Could you check a few things on this drawing? It's one solid part, dimensions in mm from its lowest x, y, z. Round coordinates to 2 decimals unless told otherwise and drop trailing zeros. Loops run counter-clockwise (first coordinate to the right, second up) from the corner with the lowest first, then second, coordinate; pieces in that order, holes last. Notation, with made-up numbers: (44, 60.25) -> (65, 60.25) arc R34 cw to (65, 90.25) -> close; hole circle Ø8 at (-29.75, 75.25). An arc over 180 degrees is marked (long way). Put each result on its own line as item: value. Start each with the question number.
1. Imagine slicing it at C-C, the plane y = 17.25. Please give me the cut outline in (x, z), and give its area (3 significant figures).
2. Imagine slicing it at D-D, the plane z = 23. Please give me the cut outline in (x, y).
3. Imagine slicing it at A-A, the plane x = 66.04. Please give me the cut outline in (y, z), and give its area (3 significant figures).
4. Imagine slicing it at B-B, the plane z = 19.05. Please give me the cut outline in (x, y), and give its area (3 significant figures).
5. I need wall thicknesses on line 1 (Z direction, x = 17.5, y = 23.25); line 2 (Z direction, x = 70.5, y = 1.5); line 3 (X direction, y = 15, z = 2). Which ranges of each line are inside material? Lowest first, please. Write a range as [from, to].
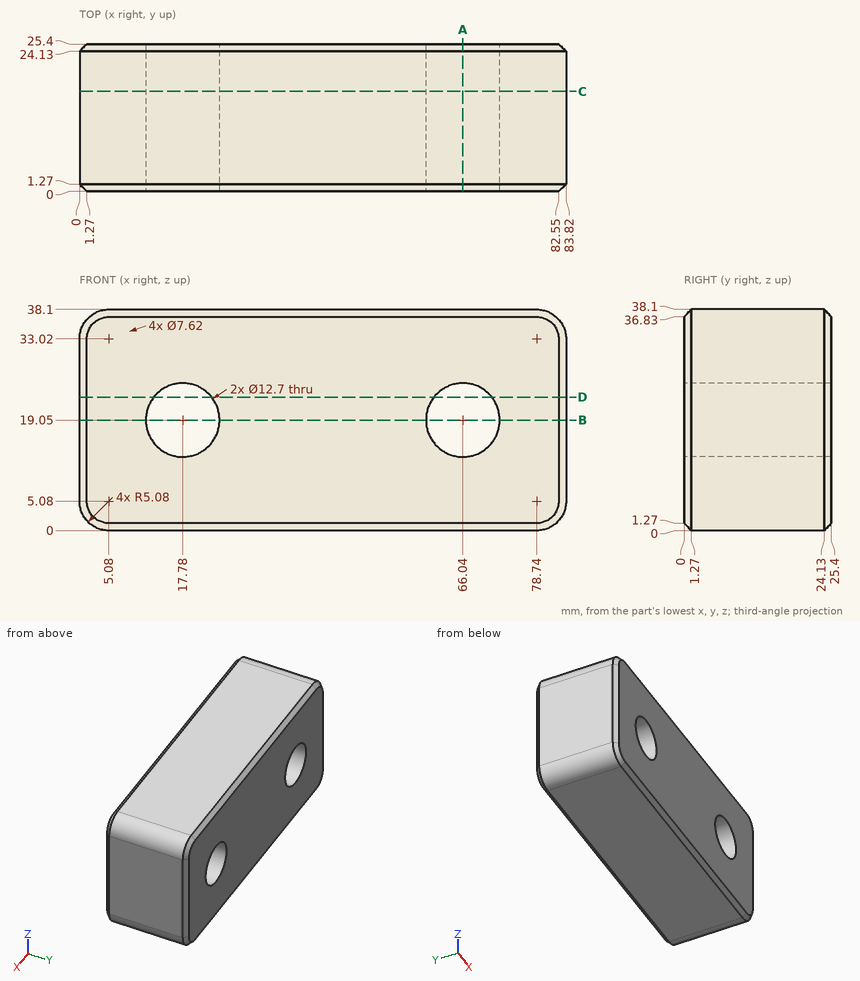
Entries:
1. outline: (0, 5.08) arc R5.08 ccw to (5.08, 0) -> (78.74, 0) arc R5.08 ccw to (83.82, 5.08) -> (83.82, 33.02) arc R5.08 ccw to (78.74, 38.1) -> (5.08, 38.1) arc R5.08 ccw to (0, 33.02) -> close; hole circle Ø12.7 at (17.78, 19.05); hole circle Ø12.7 at (66.04, 19.05)
1. area: 2,920 mm^2
2. outline: (0, 1.27) -> (1.27, 0) -> (12.81, 0) -> (12.81, 25.4) -> (1.27, 25.4) -> (0, 24.13) -> close; (22.75, 0) -> (61.07, 0) -> (61.07, 25.4) -> (22.75, 25.4) -> close; (71.01, 0) -> (82.55, 0) -> (83.82, 1.27) -> (83.82, 24.13) -> (82.55, 25.4) -> (71.01, 25.4) -> close
3. outline: (0, 1.27) -> (1.27, 0) -> (24.13, 0) -> (25.4, 1.27) -> (25.4, 12.7) -> (0, 12.7) -> close; (0, 25.4) -> (25.4, 25.4) -> (25.4, 36.83) -> (24.13, 38.1) -> (1.27, 38.1) -> (0, 36.83) -> close
3. area: 642 mm^2
4. outline: (0, 1.27) -> (1.27, 0) -> (11.43, 0) -> (11.43, 25.4) -> (1.27, 25.4) -> (0, 24.13) -> close; (24.13, 0) -> (59.69, 0) -> (59.69, 25.4) -> (24.13, 25.4) -> close; (72.39, 0) -> (82.55, 0) -> (83.82, 1.27) -> (83.82, 24.13) -> (82.55, 25.4) -> (72.39, 25.4) -> close
4. area: 1,480 mm^2
5. line 1: [0, 12.71], [25.39, 38.1]
5. line 2: [0, 14.53], [23.57, 38.1]
5. line 3: [1.04, 82.78]
